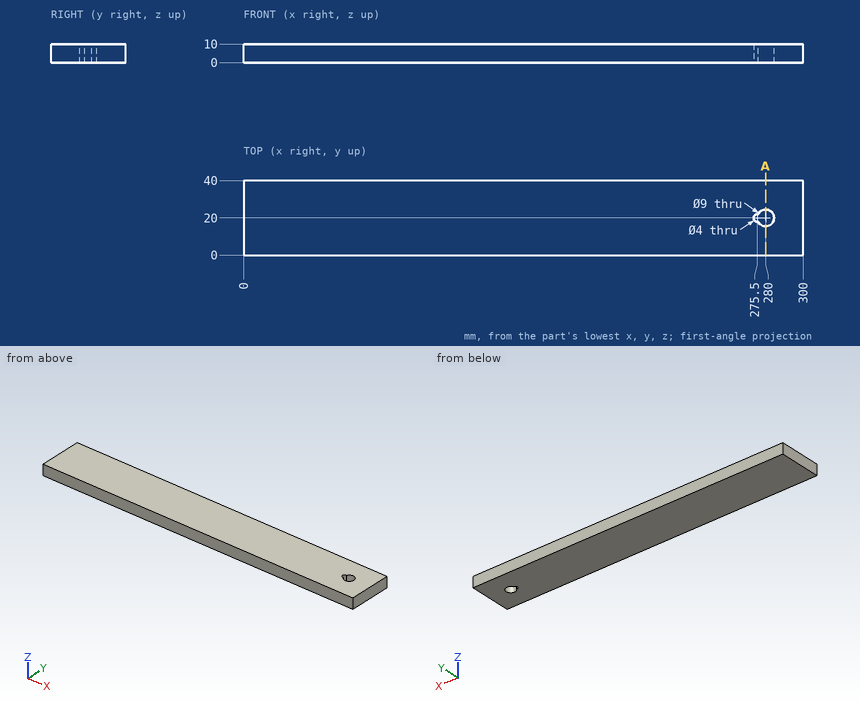
Here's the drawing with two shaded views (mm, measured from the low corner). I have some questions. Coordinates: 2 decimals unless noted, no trailing zeros. Write each loop counter-clockwise with the first axis right and the second up, starting at its lowest first coordinate (ties: lowest second). Pieces come first, ordered by that corner, then holes. Notation, with made-up numbers: (41.25, 9) -> (57.25, 9) arc R11 cw to (57.25, 17) -> close; hole circle Ø9 at (-39, -33). An arc over 180 degrees is marked (long way). One line per question, with ' | ' between items. Start each with the question number.
1. Will this pin go through, and if not, where does the flat tip stop? P1, Ø3.5, axis at x = 275.5, y = 20, coming from the -Z side.
2. Please list where these lines run through material, in increasing order: line 1 along X through (y, z) = (20, 3.5); line 2 along Y through (x, z) = (275.5, 3); line 3 along Y through (x, z) = (280, 7).
3. If we section it at A-A (x = 280): Please give me the cut outline in (y, z).
Return value:
1) P1: passes through
2) line 1: x = 0 to 273.5, 284.5 to 300 | line 2: y = 0 to 18, 22 to 40 | line 3: y = 0 to 15.5, 24.5 to 40
3) outline: (0, 0) -> (15.5, 0) -> (15.5, 10) -> (0, 10) -> close; (24.5, 0) -> (40, 0) -> (40, 10) -> (24.5, 10) -> close
